from build123d import *

# Parameters (mm, degrees)
F0_W      = 127
F0_H      = 127
F1_DEPTH  = 25.4
F3_DEPTH  = 25.4
F5_DEPTH  = 25.4
F7_DEPTH  = 25.4
F8_R      = 15.875
F9_DEPTH  = 25.4
F11_DEPTH = 25.4
F13_DEPTH = 25.4
F15_DEPTH = 25.4


with BuildPart() as f1:
    # F0 (on Top) → F1 (new body)
    with BuildSketch(Plane.XY):
        with Locations((-6.4998464659, 17.2889307044)):
            Rectangle(F0_W, F0_H)
    extrude(amount=F1_DEPTH)

    # F2 (on face) → F3 (join)
    with BuildSketch(Plane.XY.offset(25.4)):
        Polygon((-69.9998464659, 80.7889307044), (-19.1998464659, 80.7889307044), (-87.8500497752, 137.2721988958), (-138.6500497752, 137.2721988958), (-138.6500497752, 86.4721988958), (-69.9998464659, 29.9889307044), align=None)
        with BuildLine():
            ThreePointArc((-109.5878779442, 92.8645576236), (-127.335300057, 93.7629034767), (-126.8113794505, 111.5253223468))
            ThreePointArc((-126.8113794505, 111.5253223468), (-126.4226968944, 111.8842534225), (-126.0194023679, 112.2266846875))
            Line((-126.0194023679, 112.2266846875), (-110.7193396489, 125.7761775168))
            ThreePointArc((-110.7193396489, 125.7761775168), (-97.0861443246, 127.8491270452), (-89.5994854861, 116.268493473))
            ThreePointArc((-89.5994854861, 116.268493473), (-90.7041997852, 111.087822714), (-93.8261547008, 106.8084371623))
            Line((-93.8261547008, 106.8084371623), (-109.5878779442, 92.8645576236))
        make_face(mode=Mode.SUBTRACT)
    extrude(amount=-F3_DEPTH)

    # F4 (on face) → F5 (join)
    with BuildSketch(Plane.XY.offset(25.4)):
        Polygon((-19.1998464659, -46.2110692956), (-69.9998464659, -46.2110692956), (-69.9998464659, 4.5889307044), (-137.9625790448, -52.7196810429), (-137.9625790448, -103.5196810429), (-87.1625790448, -103.5196810429), align=None)
        with BuildLine():
            ThreePointArc((-124.8913826642, -77.2612392483), (-125.8684271298, -59.289751867), (-107.8930110557, -58.387869642))
            Line((-107.8930110557, -58.387869642), (-93.478630305, -71.4798248269))
            ThreePointArc((-93.478630305, -71.4798248269), (-92.3018338966, -72.4272635432), (-91.2458718834, -73.5077422033))
            ThreePointArc((-91.2458718834, -73.5077422033), (-88.9421307344, -77.38777287), (-88.1404826535, -81.8284058891))
            ThreePointArc((-88.1404826535, -81.8284058891), (-96.3332021363, -93.7016709135), (-110.3411790849, -90.2561438606))
            Line((-110.3411790849, -90.2561438606), (-124.8913826642, -77.2612392483))
        make_face(mode=Mode.SUBTRACT)
    extrude(amount=-F5_DEPTH)

    # F6 (on face) → F7 (join)
    with BuildSketch(Plane.XY.offset(25.4)):
        with BuildLine():
            Line((-86.9905296106, -9.7382222324), (-69.9998464659, 4.5889307044))
            Line((-69.9998464659, 4.5889307044), (-69.9998464659, 29.9889307044))
            Line((-69.9998464659, 29.9889307044), (-86.9905296106, 43.9683403282))
            ThreePointArc((-86.9905296106, 43.9683403282), (-102.6121797634, 17.1150590479), (-86.9905296106, -9.7382222324))
        make_face()
    extrude(amount=-F7_DEPTH)

    # F8 (on face) → F9 (cut)
    with BuildSketch(Plane.XY.offset(25.4)):
        with Locations((-71.7212476412, 17.1150590479)):
            Circle(F8_R)
    extrude(amount=-F9_DEPTH, mode=Mode.SUBTRACT)

    # F10 (on face) → F11 (join)
    with BuildSketch(Plane.XY.offset(25.4)):
        Polygon((6.2001535341, 80.7889307044), (57.0001535341, 80.7889307044), (57.0001535341, 29.9889307044), (126.4214329, 85.5217675778), (126.4214329, 136.3217675778), (75.6214329, 136.3217675778), align=None)
        with BuildLine():
            ThreePointArc((76.5939625601, 106.3933075608), (80.5762417258, 123.917512433), (98.0957891705, 119.9147932213))
            Line((98.0957891705, 119.9147932213), (109.2649622488, 102.7253014109))
            ThreePointArc((109.2649622488, 102.7253014109), (110.7921511376, 99.4142259228), (111.3155970742, 95.8056900505))
            ThreePointArc((111.3155970742, 95.8056900505), (96.237535273, 83.330321436), (86.8061762759, 100.4776896661))
            ThreePointArc((86.8061762759, 100.4776896661), (81.1206145534, 102.0919953506), (76.7813723772, 106.1047964024))
            ThreePointArc((76.7813723772, 106.1047964024), (76.6866904713, 106.2484173479), (76.5939625601, 106.3933075608))
        make_face(mode=Mode.SUBTRACT)
    extrude(amount=-F11_DEPTH)

    # F12 (on face) → F13 (cut)
    with BuildSketch(Plane.XY.offset(25.4)):
        with BuildLine():
            Line((-19.1998464659, 80.7889307044), (6.2001535341, 80.7889307044))
            Line((6.2001535341, 80.7889307044), (23.852505554, 94.9097477523))
            ThreePointArc((23.852505554, 94.9097477523), (-6.2549458696, 107.6316508681), (-36.3623972932, 94.9097477523))
            Line((-36.3623972932, 94.9097477523), (-19.1998464659, 80.7889307044))
        make_face()
    extrude(amount=-F13_DEPTH, mode=Mode.SUBTRACT)

    # F14 (on face) → F15 (cut)
    with BuildSketch(Plane.XY.offset(25.4)):
        with BuildLine():
            Line((76.7843086706, 106.1004093518), (86.8061762759, 91.133690435))
            ThreePointArc((86.8061762759, 91.133690435), (85.9155970742, 95.8056900505), (86.8061762759, 100.4776896661))
            ThreePointArc((86.8061762759, 100.4776896661), (81.1229163803, 102.0907036074), (76.7843086706, 106.1004093518))
        make_face()
    extrude(amount=-F15_DEPTH, mode=Mode.SUBTRACT)


solid = f1.part
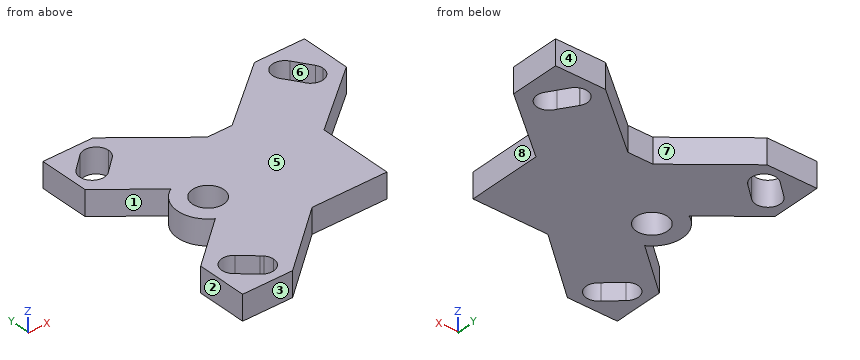
Input: part model. Units: mm. Frame: model coordinates. Face numbers are marked on the shaded views. A direction names the side the tool comes from. Coordinates: 2 decimals unless noted, no trailing zeros. Order: outer loops, then holes, each group sorted by start corner. A loop starts at its lowest first (then second) coordinate and runs counter-clockwise, first axis right, second up. Notation, with made-up numbers: M -16.5,85 L 5.5,85 A24 cw 5.5,109 Z; hole C -23.5,30 d2. An arc over 180 degrees is marked long. Write item = value, one per line. Start each with the question number.
(1) Reachability of the marked faces 4, 5, 6, 7 and 8 from +Z, -Z, +X, -X, +Y, -Y: full face, straight path, thin tool, end or side. Return the list, or none.
(2) Section A-A on y = 99. Output: boundary loops of the cut face in (x, z), and give its area (3 significant figures).
(3) Line query: line 1 along X through (y, z) = (123.5, 1.5); line 2 along X through (y, z) = (116.5, 1.5); line 3 along Y through (x, z) = (-18, 6.75). Output: solid intervals per line, ascending. Write a range as [from, to].
(4) Pull-direction query (Y, two-part tool) for the marked faces 1, 2 and 3; classes: released by +Y, released by -Y, zero draft, split by the parting line, or undercut.
(5) Section B-B on y = 9. Output: boundary loops of the cut face in (x, z), and give its area (3 significant figures).
(6) First-contact query: P1, Ø5, axis at y = 66, z = 8.5, coming from the -X side; P2, Ø5, axis at x = -22.5, z = 21, coming from the +Y side; P3, Ø7.5, axis at x = 21.5, z = 12.5, coming from the -Y side. Flat tips, straight axial feed; report the tip coordinate or a pass-through.
(7) Section D-D on z = 8.5. Give the number of separate pieces and of enclosed holes in the cut face, and give its area (3 significant figures).
(8) Section C-C on x = 0.5. Output: boundary loops of the cut face in (y, z).
Result set:
q1.face_4 = +Z, -Z, +X, +Y
q1.face_5 = +Z, +X, -X, +Y, -Y
q1.face_6 = +Z, -Z
q1.face_7 = +Z, -Z, +Y
q1.face_8 = +Z, -Z, +X, -Y
q2.outline = M -138.65,0 L -130.25,0 L -130.25,25.4 L -138.65,25.4 Z; M -102.65,0 L -41.33,0 L -41.33,25.4 L -102.65,25.4 Z; M 28.97,0 L 81.54,0 L 81.54,25.4 L 28.97,25.4 Z; M 110.91,0 L 126.42,0 L 126.42,25.4 L 110.91,25.4 Z
q2.area = 3,500 mm²
q3.line_1 = [-138.65, -113.29], [-91.86, -71.11], [59.59, 79.95], [94.72, 126.42]
q3.line_2 = [-138.65, -121.19], [-89.6, -62.6], [50.84, 75.08], [100.31, 126.42]
q3.line_3 = [-46.21, 80.79]
q4.face_1 = undercut
q4.face_2 = zero draft
q4.face_3 = released by -Y
q5.outline = M -101.53,0 L -85.37,0 L -85.37,25.4 L -101.53,25.4 Z; M -58.08,0 L 57,0 L 57,25.4 L -58.08,25.4 Z
q5.area = 3,330 mm²
q6.P1 = -116.81
q6.P2 = 85.56
q6.P3 = -46.21
q7.separate_pieces = 1
q7.enclosed_holes = 4
q7.area = 32,600 mm²
q8.outline = M -46.21,0 L 80.79,0 L 80.79,25.4 L -46.21,25.4 Z
